Input: dimensioned drawing with shaded views. Units: mm. Origin: part minimum x, y, z. A direction names the side the tool comes from. Give positions to 0.01 mm unless a question says otherwise; leave off trailing zeros. Write each loop counter-clockwise with the first axis right and the second up, starting at its lowest first coordinate (ties: lowest second). Pieces come first, ordered by that corner, then holes. Notation, with made-up numbers: M 4.25,-11.75 L 57.25,-11.75 A24 cw 57.25,19.25 Z; hole C -18.5,-35 d5. An arc over 180 degrees is marked long. Use CSV: the item, a comma, the result in double quotes. Start each with the question number.
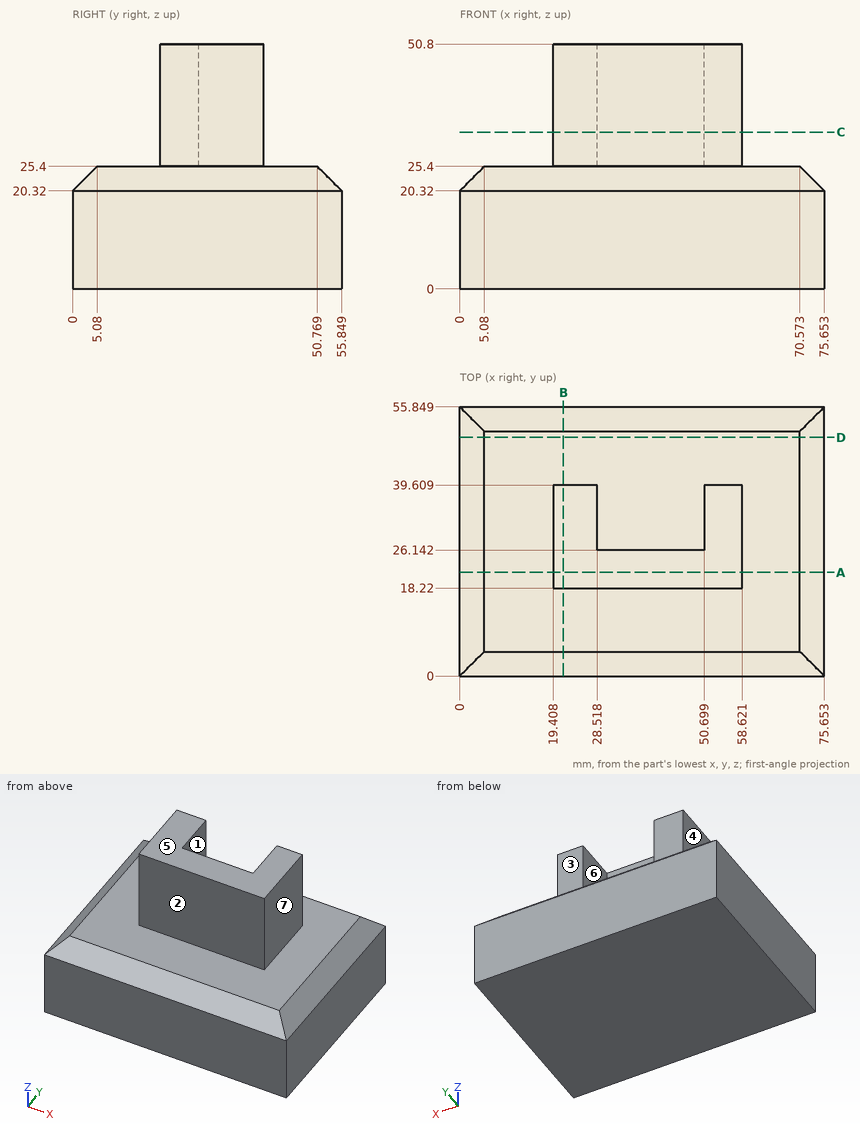
Item 1: Material intervals for probe 1 along X at (y, z) = (33.5, 27.5); probe 2 along Z at (x, y) = (6, 12); probe 3 along Y at (x, z) = (24, 36.5), sorted ascending.
Item 2: Set-up query: the marked faces 1, 2 and 3. Return all of +Z, -Z, +X, -X, +Y, -Y with unobstructed straight access to the full face (end or side cutting, diameter ignored); none if empty.
Item 3: Section C-C (z = 32.5). Return the cut outline in (x, y).
Item 4: Section A-A (y = 21.5). Return the cut outline in (x, z), plus the area to 3 significant figures.
Item 5: Contact query for flat-ended pins moving along their axis: pin 1 Ø6.5 at (x, z) = (56, 39) entering from +Y; pin 2 Ø12 at (y, z) = (8, 39.5) entering from +X; pin 3 Ø10 at (x, y) = (53, 9.5) entering from +Z; pin 4 Ø1.5 at (x, z) = (21.5, 40) entering from -Y. Output: stop coordinate, or through.
Item 6: Section B-B (x = 21.5). Return the cut outline in (y, z).
Item 7: Pull-direction query (X, two-part tool) for the marked faces 4, 5, 6 and 7; classes: released by +X, released by -X, zero draft, split by the parting line, or undercut.
Item 8: Section D-D (y = 49.5). Return the cut outline in (x, z).
Output values:
1,probe 1,"x = 19.41 to 28.52, 50.7 to 58.62"
1,probe 2,"z = 0 to 25.4"
1,probe 3,"y = 18.22 to 39.61"
2,face 1,"+Z, +Y"
2,face 2,"+Z, +X, -X, -Y"
2,face 3,"+Z, +X, -X, +Y"
3,outline,"M 19.41,18.22 L 58.62,18.22 L 58.62,39.61 L 50.7,39.61 L 50.7,26.14 L 28.52,26.14 L 28.52,39.61 L 19.41,39.61 Z"
4,outline,"M 0,0 L 75.65,0 L 75.65,20.32 L 70.57,25.4 L 58.62,25.4 L 58.62,50.8 L 19.41,50.8 L 19.41,25.4 L 5.08,25.4 L 0,20.32 Z"
4,area,"2,890 mm2"
5,pin 1,"stops at y = 39.61"
5,pin 2,"passes through"
5,pin 3,"stops at z = 25.4"
5,pin 4,"stops at y = 18.22"
6,outline,"M 0,0 L 55.85,0 L 55.85,20.32 L 50.77,25.4 L 39.61,25.4 L 39.61,50.8 L 18.22,50.8 L 18.22,25.4 L 5.08,25.4 L 0,20.32 Z"
7,face 4,"released by -X"
7,face 5,"zero draft"
7,face 6,"undercut"
7,face 7,"released by +X"
8,outline,"M 0,0 L 75.65,0 L 75.65,20.32 L 70.57,25.4 L 5.08,25.4 L 0,20.32 Z"
